For this review, take the finished solid that the model builds, in its own axes (mm). Give positions to 0.01 mm unless a question says otherwise; leave off trailing zeros. Order: outer loops, then holes, each group sorted by start corner. A loop starts at its lowest first (then second) coordinate and runs counter-clockwise, first axis right, second up.
from build123d import *

# Parameters (mm, degrees)
F0_W     = 28
F0_H     = 280
F1_DEPTH = 1035.5
F2_R     = 110
F2_R_2   = 70
F2_R_3   = 35
F3_DEPTH = 50


with BuildPart() as f1:
    # F0 (on Top) → F1 (new body)
    with BuildSketch(Plane.XY):
        Rectangle(F0_W, F0_H)
    extrude(amount=F1_DEPTH)

    # F2 (on Right) → F3 (cut, symmetric)
    with BuildSketch(Plane.YZ):
        with Locations((0, 320)):
            Circle(F2_R)
        with Locations((0, 560)):
            Circle(F2_R_2)
        with Locations((0, 760)):
            Circle(F2_R_2)
        with Locations((0, 930)):
            Circle(F2_R_3)
    extrude(amount=F3_DEPTH, both=True, mode=Mode.SUBTRACT)


solid = f1.part
1) Draft analysis for pull direction Z (two halves, no side actions). For faces 1 (the face through (14, 60, 511)), 2 (the face through (0, 2, 1035.5)), 3 (the face through (0.196, -14.32, 429.064)), state which applies: +Z half, -Z half, draft (parallel to the pull), parting line (faces both ways), or undercut.
Answer sheet:
face 1: draft
face 2: +Z half
face 3: undercut
2) We need section C-C on x = -9.5. Give the boundary of the cut face in (y, z).
Answer sheet:
outline: (-140, 0) - (140, 0) - (140, 1035.5) - (-140, 1035.5) - close; hole circle Ø220 at (0, 320); hole circle Ø140 at (0, 560); hole circle Ø140 at (0, 760); hole circle Ø70 at (0, 930)
3) We need section B-B on y = 0. Give the boundary of the cut face in (x, z).
Answer sheet:
outline: (-14, 0) - (14, 0) - (14, 210) - (-14, 210) - close; (-14, 430) - (14, 430) - (14, 490) - (-14, 490) - close; (-14, 630) - (14, 630) - (14, 690) - (-14, 690) - close; (-14, 830) - (14, 830) - (14, 895) - (-14, 895) - close; (-14, 965) - (14, 965) - (14, 1035.5) - (-14, 1035.5) - close
4) To check wall thickness, follow line 1 (Z direction, x = -0.5, y = 0); line 2 (Y direction, x = 6.75, z = 560); line 3 (Z direction, x = 2.25, y = -43.5). State the ranges of each line that lie inside material, in increasing order.
Answer sheet:
line 1: z = 0 to 210, 430 to 490, 630 to 690, 830 to 895, 965 to 1035.5
line 2: y = -140 to -70, 70 to 140
line 3: z = 0 to 218.97, 421.03 to 505.16, 614.84 to 705.16, 814.84 to 1035.5
5) We need section D-D on y = 83.5. Give the boundary of the cut face in (x, z), then the cut area to 3 significant figures.
Answer sheet:
outline: (-14, 0) - (14, 0) - (14, 248.39) - (-14, 248.39) - close; (-14, 391.61) - (14, 391.61) - (14, 1035.5) - (-14, 1035.5) - close
area: 25,000 mm2
6) We need section A-A on z = 609. Give the boundary of the cut face in (x, y).
Answer sheet:
outline: (-14, -140) - (14, -140) - (14, -49.99) - (-14, -49.99) - close; (-14, 49.99) - (14, 49.99) - (14, 140) - (-14, 140) - close
